Can you work these out from the model? Positions are in its coordinate system, mm. A direction names the side the tool comes from. Coordinates: 2 decimals unless noted, no trailing zeros. Order: outer loops, then holes, each group sorted by start corner. A loop starts at its lowest first (then second) coordinate and runs counter-clockwise, first axis right, second up.
```python
from build123d import *

# Parameters (mm, degrees)
SKETCH1_R           = 2.2225
SKETCH1_W           = 3.2004
SKETCH1_H           = 3.2004
BOSS_EXTRUDE1_DEPTH = 1.1684
SKETCH2_R           = 1.7145
CUT_EXTRUDE1_DEPTH  = 2.54


with BuildPart() as part:
    # Sketch1 → Boss-Extrude1 (new body)
    with BuildSketch(Plane.XZ):
        Polygon((33.401, -12.573), (35.56, -10.414), (35.56, -2.159), (33.401, 0), (2.159, 0), (0, -2.159), (0, -10.414), (2.159, -12.573), align=None)
        with Locations((5.08, -6.2865)):
            Circle(SKETCH1_R, mode=Mode.SUBTRACT)
        with Locations((30.48, -6.2865)):
            Circle(SKETCH1_R, mode=Mode.SUBTRACT)
        with Locations((23.495, -6.2865)):
            Rectangle(SKETCH1_W, SKETCH1_H, mode=Mode.SUBTRACT)
        with Locations((12.065, -6.2865)):
            Rectangle(SKETCH1_W, SKETCH1_H, mode=Mode.SUBTRACT)
        with Locations((17.78, -6.2865)):
            Rectangle(SKETCH1_W, SKETCH1_H, mode=Mode.SUBTRACT)
    extrude(amount=-BOSS_EXTRUDE1_DEPTH)

    # Sketch2 → Cut-Extrude1 (cut)
    with BuildSketch(Plane(origin=(0, 1.1684, 0), x_dir=(1, 0, 0), z_dir=(0, 1, 0))):
        with Locations((12.065, 6.2865)):
            Circle(SKETCH2_R)
        with Locations((17.78, 6.2865)):
            Circle(SKETCH2_R)
        with Locations((23.495, 6.2865)):
            Circle(SKETCH2_R)
    extrude(amount=-CUT_EXTRUDE1_DEPTH, mode=Mode.SUBTRACT)


solid = part.part
```
1. On a 3-axis mill with a long thin cutter (end or side, diameter ignored), from which of +Z, -Z, +X, -X, +Y, -Y can I reach the whole of each face in a straight line? I mean faces 1 (the flat face through (19.38, 1, -5)), 2 (the flat face through (18, 1, 0)). Say none if no direction works.
Completed:
face 1: +Y, -Y
face 2: +Z, +X, -X, +Y, -Y
2. Imagine slicing it at A-A on x = 5.08. Please give me the cut outline in (y, z).
Completed:
outline: (0, -12.57) - (1.17, -12.57) - (1.17, -8.51) - (0, -8.51) - close; (0, -4.06) - (1.17, -4.06) - (1.17, 0) - (0, 0) - close
3. Imagine slicing it at D-D on y = 0.7. Give the number of separate pieces and of enclosed holes in the cut face, then the cut area to 3 significant figures.
Completed:
separate pieces: 1
enclosed holes: 5
area: 375 mm2
4. I'm going to push a flat-ended pin straight in: pin 1 (3.5 mm diameter, centred on x = 5.08, z = -6.29, fed in from +Y). Where does the tip first touch, or does it pass through?
Completed:
pin 1: passes through
5. Please list where these lines run through material, in increasing order: probe 1 along X at (y, z) = (0.1, -5.75); probe 2 along Z at (x, y) = (12, 1); probe 3 along Z at (x, y) = (25, 0.25).
Completed:
probe 1: x = 0 to 2.92, 7.24 to 10.44, 13.69 to 16.15, 19.41 to 21.87, 25.12 to 28.32, 32.64 to 35.56
probe 2: z = -12.57 to -8, -4.57 to 0
probe 3: z = -12.57 to -7.89, -4.69 to 0
6. Thinking about a two-plate mould opening in X: for faces 3 (the flat face through (18, 1, -12.573)), 4 (the cylindrical face through (10.35, 0.59, -6.3)), 5 (the flat face through (21.895, 1, -5)), which applies, pulls with the +X half, pulls with the -X half, needs draft (parallel to the pull), parting line crosses it, or undercut?
Completed:
face 3: needs draft
face 4: undercut
face 5: undercut
7. Imagine slicing it at C-C on z = -11.75. Please give me the cut outline in (x, y).
Completed:
outline: (1.34, 0) - (34.22, 0) - (34.22, 1.17) - (1.34, 1.17) - close
8. Imagine slicing it at B-B on x = 12. Please give me the cut outline in (y, z).
Completed:
outline: (0, -12.57) - (1.17, -12.57) - (1.17, -8) - (0, -8) - close; (0, -4.57) - (1.17, -4.57) - (1.17, 0) - (0, 0) - close
